Solid Edge part; units mm, degrees
sketch "Sketch1" plane through (0, 0, 0) normal (0, 0, 1) x (1, 0, 0)
  circle A0 centre (6.5, 6.5) radius 6.5
extrude "ProtrusiónExtruida_3" add sketch "Sketch1" along normal blind 6.5
sketch "Sketch2" plane through (6.5, 0, 0) normal (1, 0, 0) x (0, 1, 0)
  line L0 (3.5, 6.5) -> (6.5, 6.5)
  line L1 (6.5, 1) -> (6.5, 6.5)
  line L2 (3.5, 1) -> (6.5, 1)
  line L3 (3.5, 1) -> (2.6811, 3.25)
  line L4 (3.5, 5.5) -> (2.6811, 3.25)
  line L5 (3.5, 5.5) -> (3.5, 6.5)
revolve "RevolvedCutout1" cut sketch "Sketch2" angle 360 about axis through (6.5, 6.5, 1) along (0, 0, 1)
chamfer "Chaflán_40" distance 1.5 angle 45 2 edges at (0, 6.5, 6.5) (0, 6.5, 0)
chamfer "Chaflán_41" distance 0.75 angle 45 1 edges at (6.5, 3.5, 6.5)
Model file for the job. Use its own axes, mm. Give positions to 0.01 mm unless a question says otherwise; leave off trailing zeros. Loops run counter-clockwise (first coordinate to the right, second up) from the corner with the lowest first, then second, coordinate; pieces in that order, holes last.
1) Wall check: line 1 (X direction, y = 6.5, z = 5.7); line 2 (X direction, y = 6.75, z = 4.25); line 3 (Y direction, x = 6.5, z = 1.25). Give the ranges that are in metal, low to high.
2) Saw through at C-C (z = 3). Write the cut outline in (x, y), plus the area to 3 significant figures.
3) Saw through at A-A (x = 6.5). Write the cut outline in (y, z).
4) Saw through at D-D (z = 4). Write the cut outline in (x, y).
5) Pull direction Z, two halves, no side cores. Call faces 1 (the flat face through (6, 7, 0)), 2 (the conical face through (8.357, 8.921, 5.359)), 3 (the flat face through (7, 7, 1)), 4 (the conical face through (4.643, 8.921, 1.141)): +Z half, -Z half, draft (parallel to the pull), parting line (faces both ways), or undercut.
6) Flat gauge pins, fed straight in: pin 1 Ø2 at (x, z) = (3.5, 1) entering from +Y; pin 2 Ø1.8 at (x, y) = (6, 7) entering from +Z. Where does each tip first touch, or does it go through?
Answer block:
1. line 1: x = 0.7 to 3.5, 9.5 to 12.3
1. line 2: x = 0 to 3.05, 9.95 to 13
1. line 3: y = 0.25 to 3.41, 9.59 to 12.75
2. outline: circle Ø13 at (6.5, 6.5); hole circle Ø7.46 at (6.5, 6.5)
2. area: 89.1 mm2
3. outline: (0, 1.5) - (1.5, 0) - (11.5, 0) - (13, 1.5) - (13, 5) - (11.5, 6.5) - (10.25, 6.5) - (9.5, 5.75) - (9.5, 5.5) - (10.32, 3.25) - (9.5, 1) - (3.5, 1) - (2.68, 3.25) - (3.5, 5.5) - (3.5, 5.75) - (2.75, 6.5) - (1.5, 6.5) - (0, 5) - close
4. outline: circle Ø13 at (6.5, 6.5); hole circle Ø7.09 at (6.5, 6.5)
5. face 1: -Z half
5. face 2: undercut
5. face 3: +Z half
5. face 4: undercut
6. pin 1: stops at y = 12.64
6. pin 2: stops at z = 1
